Input: part model. Units: mm. Frame: model coordinates. Give positions to 0.01 mm unless a question says otherwise; leave off trailing zeros. Order: outer loops, then holes, each group sorted by start corner. A loop starts at its lowest first (then second) coordinate and runs counter-clockwise, first axis right, second up. Notation, with made-up numbers: (55, -7.5) - (70, -7.5) arc R14 cw to (70, 19.5) - close; hole circle Ø11 at (0.5, 82.25). An arc over 180 degrees is marked (long way). Use a Markdown table: item, result.
from build123d import *

# Parameters (mm, degrees)
EXTRUDE_1_DEPTH     = 5
SKETCH_2_R          = 3
CUT_EXTRUDE_1_DEPTH = 10
SKETCH_4_R          = 3
CUT_EXTRUDE_2_DEPTH = 10
SKETCH_9_R          = 3
CUT_EXTRUDE_3_DEPTH = 10


with BuildPart() as part:
    # 草图1 → 凸台-拉伸1 (new body)
    with BuildSketch(Plane.XY):
        with BuildLine():
            Line((-15.5, 27.5), (38.5, 27.5))
            ThreePointArc((38.5, 27.5), (40.621320344, 26.621320344), (41.5, 24.5))
            Line((41.5, 24.5), (41.5, -7))
            ThreePointArc((41.5, -7), (40.621320344, -9.121320344), (38.5, -10))
            Line((38.5, -10), (33.3, -10))
            Line((33.3, -10), (31.175, -10))
            Line((31.175, -10), (-8.825, -10))
            Line((-8.825, -10), (-15.5, -10))
            ThreePointArc((-15.5, -10), (-17.621320344, -9.121320344), (-18.5, -7))
            Line((-18.5, -7), (-18.5, 24.5))
            ThreePointArc((-18.5, 24.5), (-17.621320344, 26.621320344), (-15.5, 27.5))
        make_face()
    extrude(amount=EXTRUDE_1_DEPTH)

    # 草图2 → 切除-拉伸1 (cut)
    with BuildSketch(Plane.XY.offset(5)):
        with Locations((-6.17, 21.5)):
            Circle(SKETCH_2_R)
        with Locations((29.17, 21.5)):
            Circle(SKETCH_2_R)
    extrude(amount=-CUT_EXTRUDE_1_DEPTH, mode=Mode.SUBTRACT)

    # 草图4 → 切除-拉伸2 (cut)
    with BuildSketch(Plane.XY.offset(5)):
        with Locations((-5.5, 0)):
            Circle(SKETCH_4_R)
    extrude(amount=-CUT_EXTRUDE_2_DEPTH, mode=Mode.SUBTRACT)

    # 草图9 → 切除-拉伸3 (cut)
    with BuildSketch(Plane.XY.offset(5)):
        with Locations((20.56, 0.2)):
            Circle(SKETCH_9_R)
    extrude(amount=-CUT_EXTRUDE_3_DEPTH, mode=Mode.SUBTRACT)


solid = part.part
1. Mould query, pull axis Y, two halves, no side actions, for faces 1 (the face through (-17.6, -9.14, 2.46)), 2 (the face through (-17.64, 26.6, 2.46)), 3 (the face through (26.173, 21.632, 2.535)). Classes: pulls with the +Y half, pulls with the -Y half, needs draft (parallel to the pull), parting line crosses it, or undercut.
Response:
| item | result |
|---|---|
| face 1 | pulls with the -Y half |
| face 2 | pulls with the +Y half |
| face 3 | undercut |
2. Section query A-A (y = 21.5). Return loops of the section in (x, z).
Response:
| item | result |
|---|---|
| outline | (-18.5, 0) - (-9.17, 0) - (-9.17, 5) - (-18.5, 5) - close; (-3.17, 0) - (26.17, 0) - (26.17, 5) - (-3.17, 5) - close; (32.17, 0) - (41.5, 0) - (41.5, 5) - (32.17, 5) - close |
3. Material intervals for line 1 along Y through (x, z) = (-5.5, 2.45); line 2 along X through (y, z) = (1.5, 3.9); line 3 along Y through (x, z) = (29.17, 2.15), sorted ascending.
Response:
| item | result |
|---|---|
| line 1 | y = -10 to -3, 3 to 18.58, 24.42 to 27.5 |
| line 2 | x = -18.5 to -8.1, -2.9 to 17.86, 23.26 to 41.5 |
| line 3 | y = -10 to 18.5, 24.5 to 27.5 |
4. Pin query (flat end, axial travel): pin 1 (5.5 mm diameter, centred on x = 29.17, y = 21.5, fed in from -Z) (1 decimal). Return the tip coordinate at first contact, or that it passes through.
Response:
| item | result |
|---|---|
| pin 1 | passes through |
5. Section query C-C (z = 3.45). Return loops of the section in (x, y), then the cut area to 3 significant figures.
Response:
| item | result |
|---|---|
| outline | (-18.5, -7) arc R3 ccw to (-15.5, -10) - (38.5, -10) arc R3 ccw to (41.5, -7) - (41.5, 24.5) arc R3 ccw to (38.5, 27.5) - (-15.5, 27.5) arc R3 ccw to (-18.5, 24.5) - close; hole circle Ø6 at (-6.17, 21.5); hole circle Ø6 at (-5.5, 0); hole circle Ø6 at (20.56, 0.2); hole circle Ø6 at (29.17, 21.5) |
| area | 2,130 mm^2 |
6. Section query B-B (x = 20.56). Return loops of the section in (y, z), then the cut area to 4 significant figures.
Response:
| item | result |
|---|---|
| outline | (-10, 0) - (-2.8, 0) - (-2.8, 5) - (-10, 5) - close; (3.2, 0) - (27.5, 0) - (27.5, 5) - (3.2, 5) - close |
| area | 157.5 mm^2 |
7. Section query D-D (x = -5.5). Return loops of the section in (y, z), then the cut area to 3 significant figures.
Response:
| item | result |
|---|---|
| outline | (-10, 0) - (-3, 0) - (-3, 5) - (-10, 5) - close; (3, 0) - (18.58, 0) - (18.58, 5) - (3, 5) - close; (24.42, 0) - (27.5, 0) - (27.5, 5) - (24.42, 5) - close |
| area | 128 mm^2 |
